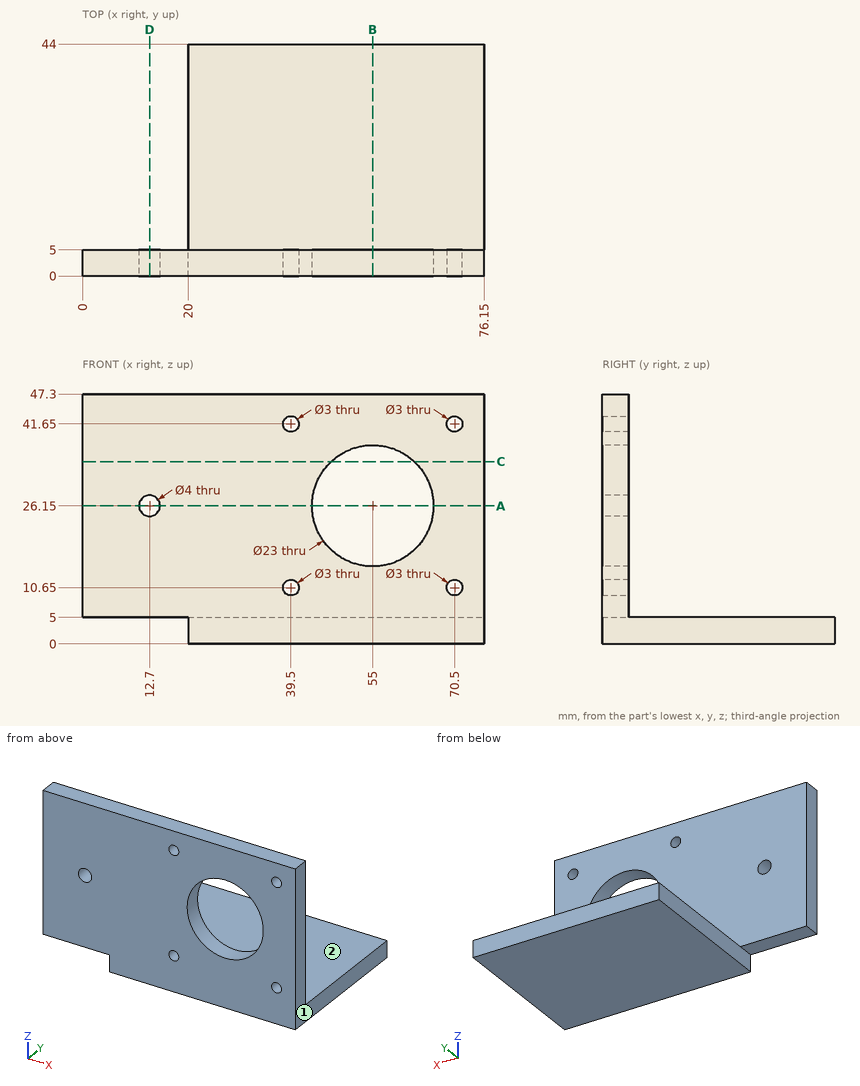
Geometry check sheet. Reference: drawing and pictorial views, mm from the part's lowest x, y, z. A direction names the side the tool comes from. Give positions to 0.01 mm unless a question says otherwise; leave off trailing zeros. Loops run counter-clockwise (first coordinate to the right, second up) from the corner with the lowest first, then second, coordinate; pieces in that order, holes last. Notation, with made-up numbers: M -7.75,42 L 5.25,42 A18 cw 5.25,53 Z; hole C 78,0.5 d1. An arc over 180 degrees is marked long. One line per question, with ' | ' between items.
Item 1: Section check B-B, the plane x = 55. Record the cut outline in (y, z).
Completed:
outline: M 0,0 L 44,0 L 44,5 L 5,5 L 5,14.65 L 0,14.65 Z; M 0,37.65 L 5,37.65 L 5,47.3 L 0,47.3 Z
Item 2: Thickness scan on line 1 (Z direction, x = 70.5, y = 1.95); line 2 (X direction, y = 3.4, z = 10.65); line 3 (Z direction, x = 55, y = 1.1). Record the ranges inside material, lowest first. Write a range as [from, to].
Completed:
line 1: z = [0, 9.15], [12.15, 40.15], [43.15, 47.3] | line 2: x = [0, 38], [41, 69], [72, 76.15] | line 3: z = [0, 14.65], [37.65, 47.3]
Item 3: Section check C-C, the plane z = 34.5. Record the cut outline in (x, y), plus the area to 3 significant figures.
Completed:
outline: M 0,0 L 47.09,0 L 47.09,5 L 0,5 Z; M 62.91,0 L 76.15,0 L 76.15,5 L 62.91,5 Z | area: 302 mm^2
Item 4: Section check A-A, the plane z = 26.15. Record the cut outline in (x, y), plus the area to 3 significant figures.
Completed:
outline: M 0,0 L 10.7,0 L 10.7,5 L 0,5 Z; M 14.7,0 L 43.5,0 L 43.5,5 L 14.7,5 Z; M 66.5,0 L 76.15,0 L 76.15,5 L 66.5,5 Z | area: 246 mm^2
Item 5: Tool access check on the marked faces 1 and 2. Record the directions out of +Z, -Z, +X, -X, +Y, -Y that give a thin tool (end or side, any length) a straight path to the whole face; none if there is none.
Completed:
face 1: +Z, -Z, +X, +Y, -Y | face 2: +Z, +X, -X, +Y
Item 6: Depth check by flat-ended pin: P1, Ø2, axis at x = 65.5, y = 22, coming from the +Z side; P2, Ø2.5, axis at x = 39.5, z = 10.65, coming from the +Y side; P3, Ø1.5, axis at y = 29, z = 1.5, coming from the -X side; P4, Ø1.5, axis at x = 11, y = 2, coming from the -Z side. Enter the tip coordinate at first touch or a pass-through.
Completed:
P1: stops at z = 5 | P2: passes through | P3: stops at x = 20 | P4: stops at z = 5
Item 7: Section check D-D, the plane x = 12.7. Record the cut outline in (y, z), plus the area to 4 significant figures.
Completed:
outline: M 0,5 L 5,5 L 5,24.15 L 0,24.15 Z; M 0,28.15 L 5,28.15 L 5,47.3 L 0,47.3 Z | area: 191.5 mm^2
